Could you check a few things on this model? Use its own coordinates, in mm. Coordinates: 2 decimals unless noted, no trailing zeros. Loops run counter-clockwise (first coordinate to the right, second up) from the corner with the lowest first, then second, coordinate; pieces in that order, holes last. Notation, with made-up numbers: (21.5, -20.75) -> (80.5, -20.75) arc R6 ccw to (80.5, -9.75) -> close; hole circle Ø11 at (58, 61.25). An arc over 180 degrees is marked (long way). One line per question, with ' | ' between items.
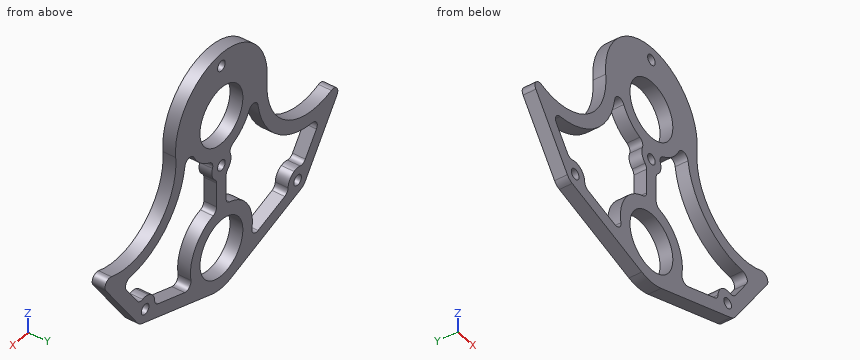
from build123d import *

# Parameters (mm, degrees)
F0_R     = 2.5527
F0_R_2   = 14.2875
F1_DEPTH = 6.35
F2_F1_R  = 3.175
F2_F2_R  = 3.175
F4_DEPTH = 25.4
F5_R     = 3.175


# Not quite as in the source:
# - a pattern or mirror of a feature is missing from the dataset's text; its kind, count and spacing are read off the source's solid


with BuildPart() as f1:
    # F0 (on Front) → F1 (new body)
    with BuildSketch(Plane.XZ):
        with BuildLine():
            ThreePointArc((-30.44415143, 64.2793510436), (-51.27863842, 31.2336995415), (-88.5449286211, 42.9518284873))
            Line((-88.5449286211, 42.9518284873), (-56.0059264265, -3.6360459351))
            ThreePointArc((-56.0059264265, -3.6360459351), (-54.5853345088, -5.0984058937), (-52.7745376605, -6.0352051355))
            Line((-52.7745376605, -6.0352051355), (-6.4172473966, -21.2019166903))
            ThreePointArc((-6.4172473966, -21.2019166903), (0, -22.225), (6.4172473966, -21.2019166903))
            Line((6.4172473966, -21.2019166903), (52.7745376605, -6.0352051355))
            ThreePointArc((52.7745376605, -6.0352051355), (54.5853345088, -5.0984058937), (56.0059264265, -3.6360459351))
            Line((56.0059264265, -3.6360459351), (88.5449286211, 42.9518284873))
            ThreePointArc((88.5449286211, 42.9518284873), (51.27863842, 31.2336995415), (30.44415143, 64.2793510436))
            ThreePointArc((30.44415143, 64.2793510436), (0, 97.7265), (-30.44415143, 64.2793510436))
        make_face()
        with Locations((-50.8, 0)):
            Circle(F0_R, mode=Mode.SUBTRACT)
        with Locations((0, -1.5875)):
            Circle(F0_R_2, mode=Mode.SUBTRACT)
        with Locations((50.8, 0)):
            Circle(F0_R, mode=Mode.SUBTRACT)
        with Locations((0, 40.5765)):
            Circle(F0_R, mode=Mode.SUBTRACT)
        with Locations((0, 65.9765)):
            Circle(F0_R_2, mode=Mode.SUBTRACT)
        with Locations((0, 91.3765)):
            Circle(F0_R, mode=Mode.SUBTRACT)
    extrude(amount=F1_DEPTH)

    # F2: fillet of radius 3.175 on 2 edges, made by hand

    # F2_f1
    f2_f1_edges = [f1.edges().sort_by_distance(p)[0] for p in [
        (-88.5449286211, -3.175, 42.9518284873),
    ]]
    fillet(f2_f1_edges, radius=F2_F1_R)

    # F2_f2
    f2_f2_edges = [f1.edges().sort_by_distance(p)[0] for p in [
        (88.5449286211, -3.175, 42.9518284873),
    ]]
    fillet(f2_f2_edges, radius=F2_F2_R)

    # F3 (on face) → F4 (cut)
    with BuildSketch(Plane.XZ.offset(6.35)):
        with BuildLine():
            Line((3.175, 35.0772394145), (3.175, 18.8043067186))
            ThreePointArc((3.175, 18.8043067186), (18.2678223179, 8.0142224503), (18.5965200171, -10.5360110216))
            Line((18.5965200171, -10.5360110216), (44.7647958403, -1.9745379709))
            ThreePointArc((44.7647958403, -1.9745379709), (45.0527871506, 2.7003757871), (48.4675934129, 5.9061293383))
            ThreePointArc((48.4675934129, 5.9061293383), (51.5398921213, 6.306746055), (54.4360459499, 5.2059254026))
            Line((54.4360459499, 5.2059254026), (67.0131976966, 23.2133234987))
            ThreePointArc((67.0131976966, 23.2133234987), (39.0870703991, 30.7510953733), (24.3679226321, 55.6515628324))
            ThreePointArc((24.3679226321, 55.6515628324), (21.7379294481, 58.3195031239), (18.3969634882, 56.6245942764))
            ThreePointArc((18.3969634882, 56.6245942764), (12.3594159846, 49.4492121774), (3.7699852595, 45.6862654673))
            ThreePointArc((3.7699852595, 45.6862654673), (6.3400365543, 40.2209321773), (3.175, 35.0772394145))
        make_face()
    f4 = extrude(amount=-F4_DEPTH, mode=Mode.SUBTRACT)

    # F4_copies: F4 across plane
    add(f4.mirror(Plane(origin=(0, 0, 0), x_dir=(0, 0, -1), z_dir=(-1, 0, 0))), mode=Mode.SUBTRACT)

    # F5
    f5_edges = [f1.edges().sort_by_distance(p)[0] for p in [
        (3.769985, -3.175, 45.686265),
        (3.175, -3.175, 35.077239),
        (3.175, -3.175, 18.804307),
        (18.59652, -3.175, -10.536011),
        (44.764796, -3.175, -1.974538),
        (54.436046, -3.175, 5.205925),
        (67.013198, -3.175, 23.213323),
        (-3.769985, -3.175, 45.686265),
        (-67.013198, -3.175, 23.213323),
        (-54.436046, -3.175, 5.205925),
        (-44.764796, -3.175, -1.974538),
        (-18.59652, -3.175, -10.536011),
        (-3.175, -3.175, 18.804307),
        (-3.175, -3.175, 35.077239),
    ]]
    fillet(f5_edges, radius=F5_R)


solid = f1.part
1) If we section it at B-B on x = -50.8: Please give me the cut outline in (y, z).
Data:
outline: (-6.35, -6.68) -> (0, -6.68) -> (0, -2.55) -> (-6.35, -2.55) -> close; (-6.35, 2.55) -> (0, 2.55) -> (0, 6.35) -> (-6.35, 6.35) -> close; (-6.35, 24.69) -> (0, 24.69) -> (0, 31.41) -> (-6.35, 31.41) -> close
2) I need wall thicknesses on line 1 along X through (y, z) = (-1.75, 22) (3 decimals); line 2 along X through (y, z) = (-3.5, 8.5); line 3 along Z through (x, y) = (2, -1.75). Which ranges of each line are inside material? Lowest first, please. Write a range as from..to.
Data:
line 1: -73.911..-63.009, -3.175..3.175, 63.009..73.911 | line 2: -64.48..-56.74, -18..-10.12, 10.12..18, 56.74..64.48 | line 3: -22.13..-15.73, 12.56..38.99, 42.16..51.83, 80.12..89.79, 92.96..97.66
3) I'm going to push flat-ended pins straight in: pin 1 Ø3 at (x, z) = (0, 40.58) entering from -Y; pin 2 Ø3 at (y, z) = (-4, 26.5) entering from -X; pin 3 Ø2 at (y, z) = (-1.5, -5) entering from +X. Where does each tip first touch, or does it pass through?
Data:
pin 1: through | pin 2: x = -77.56 | pin 3: x = 55.73
4) If we section it at A-A on x = 0: Give the number of separate pieces and of enclosed holes in the cut face, and give its area (3 significant figures).
Data:
separate pieces: 5 | enclosed holes: 0 | area: 334 mm²
